from build123d import *

# Parameters (mm, degrees)
MAIN_DEPTH      = 100
SKETCH2_R       = 1.25
SKETCH2_R_2     = 1.5
MAINHOLES_DEPTH = 6.5
SKETCH3_W       = 1
SKETCH3_H       = 60
SKETCH3_W_2     = 4
PINHOLES_DEPTH  = 2.5


with BuildPart() as part:
    # Sketch1 → Main (new body)
    with BuildSketch(Plane.XY):
        Polygon((-5, 0), (5, 0), (5, -4.5), (1.45, -4.5), (1.45, -5.5), (-1.45, -5.5), (-1.45, -4.5), (-5, -4.5), align=None)
    extrude(amount=MAIN_DEPTH)

    # Sketch2 → MainHoles (cut, through all)
    with BuildSketch(Plane(origin=(0, 0, 0), x_dir=(1, 0, 0), z_dir=(0, 1, 0))):
        with Locations((0, -85)):
            Circle(SKETCH2_R)
        with Locations((0, -15)):
            Circle(SKETCH2_R)
        with Locations((0, -5)):
            Circle(SKETCH2_R_2)
        with Locations((0, -95)):
            Circle(SKETCH2_R_2)
    extrude(amount=-MAINHOLES_DEPTH, mode=Mode.SUBTRACT)

    # Sketch3 → PinHoles (cut)
    with BuildSketch(Plane(origin=(0, 0, 0), x_dir=(1, 0, 0), z_dir=(0, 1, 0))):
        with Locations((4.5, -50)):
            Rectangle(SKETCH3_W, SKETCH3_H)
        with Locations((0.5, -50)):
            Rectangle(SKETCH3_W_2, SKETCH3_H)
    extrude(amount=-PINHOLES_DEPTH, mode=Mode.SUBTRACT)


solid = part.part
Design review of the part built by this model. Coordinates are the model's own, in mm. A direction names the side the tool comes from. Round coordinates to 2 decimals unless told otherwise and drop trailing zeros. Order: outer loops, then holes, each group sorted by start corner. A loop starts at its lowest first (then second) coordinate and runs counter-clockwise, first axis right, second up.
1) Consider section D-D (z = 51.5). State the section outline as (x, y) points.
The answers:
outline: (-5, -4.5) - (-1.45, -4.5) - (-1.45, -5.5) - (1.45, -5.5) - (1.45, -4.5) - (5, -4.5) - (5, -2.5) - (4, -2.5) - (4, 0) - (2.5, 0) - (2.5, -2.5) - (-1.5, -2.5) - (-1.5, 0) - (-5, 0) - close
2) Consider section C-C (y = -1.15). State the section outline as (x, z) points.
The answers:
outline: (-5, 0) - (5, 0) - (5, 20) - (4, 20) - (4, 80) - (5, 80) - (5, 100) - (-5, 100) - close; hole circle Ø3 at (0, 5); hole (-1.5, 20) - (2.5, 20) - (2.5, 80) - (-1.5, 80) - close; hole circle Ø3 at (0, 95); hole circle Ø2.5 at (0, 15); hole circle Ø2.5 at (0, 85)
3) Consider section B-B (z = 15). State the section outline as (x, y) points.
The answers:
outline: (-5, -4.5) - (-1.45, -4.5) - (-1.45, -5.5) - (-1.25, -5.5) - (-1.25, 0) - (-5, 0) - close; (1.25, -5.5) - (1.45, -5.5) - (1.45, -4.5) - (5, -4.5) - (5, 0) - (1.25, 0) - close
4) For L1, parallel to Z at x = 0, y = -1.9; L2, parallel to X at y = -1.95, z = 95; L3, parallel to Z at x = 0, y = -3.15, list the stretches that pass through material, from the lowest coordinate up.
The answers:
L1: z = 0 to 3.5, 6.5 to 13.75, 16.25 to 20, 80 to 83.75, 86.25 to 93.5, 96.5 to 100
L2: x = -5 to -1.5, 1.5 to 5
L3: z = 0 to 3.5, 6.5 to 13.75, 16.25 to 83.75, 86.25 to 93.5, 96.5 to 100
5) Machinability: for faces 1 (the flat face through (0, -5.5, 98)), 2 (the flat face through (3, -4.5, 49)), 3 (the flat face through (0, -1, 80)), which of the approach directions +Z, -Z, +X, -X, +Y, -Y give a long, thin tool a straight path to every point of the face, cutting with its end or side? Answer none if there is none.
The answers:
face 1: +Z, -Z, +X, -X, -Y
face 2: +Z, -Z, +X, -Y
face 3: +Y
6) Clearance check with flat-ended pins moving along their axes: pin 1 Ø0.8 at (y, z) = (-5, 3) entering from +X; pin 2 Ø0.8 at (y, z) = (-5, 34) entering from -X; pin 3 Ø0.8 at (x, y) = (-0.5, -1) entering from -Z; pin 4 Ø1.2 at (y, z) = (-1, 44) entering from +X. State where each tip first meets the part, or that it passes through.
The answers:
pin 1: stops at x = 1.45
pin 2: stops at x = -1.45
pin 3: stops at z = 0
pin 4: stops at x = 4
7) Consider section A-A (x = 0). State the section outline as (y, z) points, plus the area to 4 significant figures.
The answers:
outline: (-5.5, 0) - (0, 0) - (0, 3.5) - (-5.5, 3.5) - close; (-5.5, 6.5) - (0, 6.5) - (0, 13.75) - (-5.5, 13.75) - close; (-5.5, 16.25) - (0, 16.25) - (0, 20) - (-2.5, 20) - (-2.5, 80) - (0, 80) - (0, 83.75) - (-5.5, 83.75) - close; (-5.5, 86.25) - (0, 86.25) - (0, 93.5) - (-5.5, 93.5) - close; (-5.5, 96.5) - (0, 96.5) - (0, 100) - (-5.5, 100) - close
area: 339.5 mm2
8) Draft analysis for pull direction Z (two halves, no side actions). For faces 4 (the cylindrical face through (1.43, -2.71, 94.55)), 5 (the flat face through (-2, 0, 49)), 6 (the flat face through (4, -1, 50)), 7 (the flat face through (0, -2, 100)), state which applies: released by +Z, released by -Z, zero draft, split by the parting line, or undercut.
The answers:
face 4: undercut
face 5: zero draft
face 6: undercut
face 7: released by +Z
